For this review, take the finished solid that the model builds, in its own axes (mm). Round coordinates to 2 decimals unless told otherwise and drop trailing zeros. Loops run counter-clockwise (first coordinate to the right, second up) from the corner with the lowest first, then second, coordinate; pieces in that order, holes last.
1. Consider section A-A on y = 0.3. State the section outline as (x, z) points, then the cut area to 3 significant figures.
2. Consider section C-C on z = -18. State the section outline as (x, y) points.
3. To check wall thickness, follow line 1 along X through (y, z) = (0.05, -5); line 2 along Z through (x, y) = (12.75, 0.05); line 3 along Z through (x, y) = (14.5, 0.4). State the ranges of each line that lie inside material, in increasing order.
4. Consider section B-B on z = 5. State the section outline as (x, y) points.
5. Clearance check with flat-ended pins moving along their axes: pin 1 Ø4.5 at (x, z) = (-37.75, -5) entering from -Y; pin 2 Ø0.8 at (x, y) = (-40.5, 0.5) entering from +Z. State where each tip first meets the part, or that it passes through.
from build123d import *

# Parameters (mm, degrees)
SKETCH1_W                                    = 5
SKETCH1_H                                    = 25
SKETCH1_W_2                                  = 25
SKETCH1_H_2                                  = 50
BOSS_EXTRUDE1_DEPTH                          = 1.5
CSK_FOR_M3_COUNTERSUNK_FLAT_HEAD_SCR_2_COUNT = 2
CSK_FOR_M3_COUNTERSUNK_FLAT_HEAD_SCR_2_PITCH = 10
CSK_FOR_M3_COUNTERSUNK_FLAT_HEAD_SCR_3_COUNT = 2
CSK_FOR_M3_COUNTERSUNK_FLAT_HEAD_SCR_3_PITCH = 51.480578862
CSK_FOR_M3_COUNTERSUNK_FLAT_HEAD_SCR_4_COUNT = 2
CSK_FOR_M3_COUNTERSUNK_FLAT_HEAD_SCR_4_PITCH = 50.5


with BuildPart() as part:
    # Sketch1 → Boss-Extrude1 (new body)
    with BuildSketch(Plane(origin=(0, 0, 0), x_dir=(1, 0, 0), z_dir=(0, 1, 0))):
        Polygon((12.5, 25), (-12.5, 25), (-12.5, -25), (12.5, -25), (12.5, -12.5), (12.5, 12.5), align=None)
        with Locations((15, 0)):
            Rectangle(SKETCH1_W, SKETCH1_H)
        with Locations((-25, 0)):
            Rectangle(SKETCH1_W_2, SKETCH1_H_2)
        with Locations((-40, 0)):
            Rectangle(SKETCH1_W, SKETCH1_H)
    extrude(amount=BOSS_EXTRUDE1_DEPTH)

    # Sketch3 → CSK for M3 Countersunk Flat Head Screw1 (revolve, cut)
    with BuildSketch(Plane(origin=(12.75, 1.5, 5), x_dir=(0, 0, 1), z_dir=(1, 0, 0))):
        Polygon((0, 0), (0, 1.5), (1.7, 1.5), (1.7, 1.45), (3.15, 0), align=None)
    csk_for_m3_countersunk_flat_head_screw1 = revolve(axis=Axis((12.75, 7.85, 5), (0, -1, 0)), mode=Mode.SUBTRACT)

    # CSK for M3 Countersunk Flat Head Scr 2: CSK for M3 Countersunk Flat Head Screw1 ×2
    with Locations(*[(0, 0, -i * CSK_FOR_M3_COUNTERSUNK_FLAT_HEAD_SCR_2_PITCH) for i in range(1, CSK_FOR_M3_COUNTERSUNK_FLAT_HEAD_SCR_2_COUNT)]):
        add(csk_for_m3_countersunk_flat_head_screw1, mode=Mode.SUBTRACT)

    # CSK for M3 Countersunk Flat Head Scr 3: CSK for M3 Countersunk Flat Head Screw1 ×2
    with Locations(*[Vector(-0.9809524507300751, 0, -0.19424801004555947) * (i * CSK_FOR_M3_COUNTERSUNK_FLAT_HEAD_SCR_3_PITCH) for i in range(1, CSK_FOR_M3_COUNTERSUNK_FLAT_HEAD_SCR_3_COUNT)]):
        add(csk_for_m3_countersunk_flat_head_screw1, mode=Mode.SUBTRACT)

    # CSK for M3 Countersunk Flat Head Scr 4: CSK for M3 Countersunk Flat Head Screw1 ×2
    with Locations(*[(-i * CSK_FOR_M3_COUNTERSUNK_FLAT_HEAD_SCR_4_PITCH, 0, 0) for i in range(1, CSK_FOR_M3_COUNTERSUNK_FLAT_HEAD_SCR_4_COUNT)]):
        add(csk_for_m3_countersunk_flat_head_screw1, mode=Mode.SUBTRACT)


solid = part.part
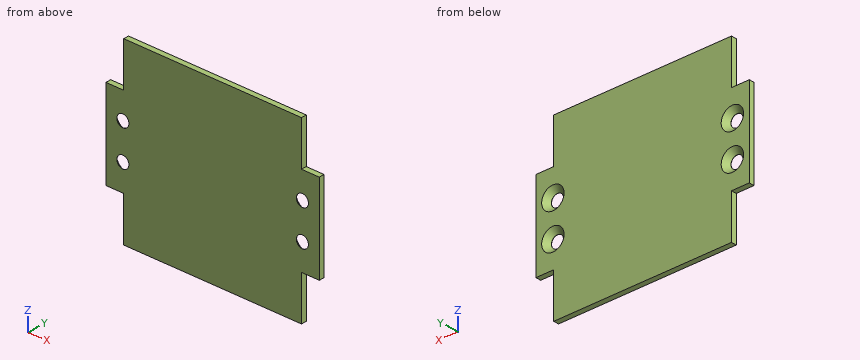
Resolved:
1. outline: (-42.5, -12.5) - (-37.5, -12.5) - (-37.5, -25) - (12.5, -25) - (12.5, -12.5) - (17.5, -12.5) - (17.5, 12.5) - (12.5, 12.5) - (12.5, 25) - (-37.5, 25) - (-37.5, 12.5) - (-42.5, 12.5) - close; hole circle Ø3.9 at (-37.75, -5); hole circle Ø3.9 at (-37.75, 5); hole circle Ø3.9 at (12.75, -5); hole circle Ø3.9 at (12.75, 5)
1. area: 2,700 mm2
2. outline: (-37.5, 0) - (12.5, 0) - (12.5, 1.5) - (-37.5, 1.5) - close
3. line 1: x = -42.5 to -39.45, -36.05 to 11.05, 14.45 to 17.5
3. line 2: z = -12.5 to -6.7, -3.3 to 3.3, 6.7 to 12.5
3. line 3: z = -12.5 to -6.07, -3.93 to 3.93, 6.07 to 12.5
4. outline: (-42.5, 0) - (-39.45, 0) - (-39.45, 0.05) - (-40.9, 1.5) - (-42.5, 1.5) - close; (-36.05, 0) - (11.05, 0) - (11.05, 0.05) - (9.6, 1.5) - (-34.6, 1.5) - (-36.05, 0.05) - close; (14.45, 0) - (17.5, 0) - (17.5, 1.5) - (15.9, 1.5) - (14.45, 0.05) - close
5. pin 1: stops at y = 0
5. pin 2: stops at z = 12.5
